Verification items for the finished model (mm, model axes). A direction names the side the tool comes from. Give positions to 0.01 mm unless a question says otherwise; leave off trailing zeros. Write each loop counter-clockwise with the first axis right and the second up, starting at its lowest first coordinate (ties: lowest second). Pieces come first, ordered by that corner, then holes.
from build123d import *

# Parameters (mm, degrees)
SKETCH1_W                                      = 223.52
SKETCH1_H                                      = 50.8
SKETCH1_R                                      = 3.2385
BOSS_EXTRUDE1_DEPTH                            = 6.858
SKETCH2_W                                      = 20
SKETCH2_H                                      = 6.35
BOSS_EXTRUDE2_DEPTH                            = 17.78
SKETCH3_R                                      = 2.25
CUT_EXTRUDE1_DEPTH                             = 17.78
SKETCH4_W                                      = 2.54
SKETCH4_H                                      = 17.78
BOSS_EXTRUDE3_DEPTH                            = 17.78
CUT_EXTRUDE2_DEPTH                             = 20
LPATTERN1_COUNT                                = 2
LPATTERN1_PITCH                                = 101.76
BOSS_EXTRUDE4_DEPTH                            = 2.54
CSK_FOR_6_FLAT_HEAD_MACHINE_SCREW1_D           = 3.7973
CSK_FOR_6_FLAT_HEAD_MACHINE_SCREW1_CSINK_D     = 7.9697834
CSK_FOR_6_FLAT_HEAD_MACHINE_SCREW1_CSINK_ANGLE = 82


with BuildPart() as part:
    # Sketch1 → Boss-Extrude1 (new body)
    with BuildSketch(Plane.XY):
        Rectangle(SKETCH1_W, SKETCH1_H)
        with Locations((-54.61, 6.35)):
            Circle(SKETCH1_R, mode=Mode.SUBTRACT)
        with Locations((54.61, 6.35)):
            Circle(SKETCH1_R, mode=Mode.SUBTRACT)
    extrude(amount=BOSS_EXTRUDE1_DEPTH)

    # Sketch2 → Boss-Extrude2 (add)
    with BuildSketch(Plane.XY.offset(6.858)):
        with Locations((-101.76, -22.225)):
            Rectangle(SKETCH2_W, SKETCH2_H)
    boss_extrude2 = extrude(amount=BOSS_EXTRUDE2_DEPTH)

    # Sketch3 → Cut-Extrude1 (cut)
    with BuildSketch(Plane(origin=(0, -19.05, 0), x_dir=(1, 0, 0), z_dir=(0, 1, 0))):
        with Locations((-101.76, -15.748)):
            Circle(SKETCH3_R)
    cut_extrude1 = extrude(amount=-CUT_EXTRUDE1_DEPTH, mode=Mode.SUBTRACT)

    # Sketch4 → Boss-Extrude3 (add)
    with BuildSketch(Plane(origin=(0, -19.05, 0), x_dir=(1, 0, 0), z_dir=(0, 1, 0))):
        with Locations((-110.49, -15.748)):
            Rectangle(SKETCH4_W, SKETCH4_H)
        with Locations((-93.03, -15.748)):
            Rectangle(SKETCH4_W, SKETCH4_H)
    boss_extrude3 = extrude(amount=BOSS_EXTRUDE3_DEPTH)

    # Sketch6 → Cut-Extrude2 (cut)
    with BuildSketch(Plane.ZY.offset(111.76)):
        Polygon((24.638, -1.27), (6.858, -1.27), (24.638, -19.05), align=None)
    cut_extrude2 = extrude(amount=-CUT_EXTRUDE2_DEPTH, mode=Mode.SUBTRACT)

    # LPattern1: Boss-Extrude2, Cut-Extrude1, Boss-Extrude3, Cut-Extrude2 ×2
    with Locations(*[(i * LPATTERN1_PITCH, 0, 0) for i in range(1, LPATTERN1_COUNT)]):
        add(boss_extrude2)
        add(cut_extrude1, mode=Mode.SUBTRACT)
        add(boss_extrude3)
        add(cut_extrude2, mode=Mode.SUBTRACT)

    # Sketch7 → Boss-Extrude4 (add)
    with BuildSketch(Plane.ZY.offset(111.76)):
        Polygon((24.638, -19.05), (24.638, 25.4), (6.858, 25.4), (6.858, -1.27), align=None)
    extrude(amount=-BOSS_EXTRUDE4_DEPTH)

    # CSK for #6 Flat Head Machine Screw1 (through all)
    with Locations(Plane(origin=(0, 0, 0), x_dir=(-1, 0, 0), z_dir=(0, 0, -1))):
        with Locations((-105.41, 12.7), (-105.41, -12.7)):
            CounterSinkHole(CSK_FOR_6_FLAT_HEAD_MACHINE_SCREW1_D / 2, CSK_FOR_6_FLAT_HEAD_MACHINE_SCREW1_CSINK_D / 2, counter_sink_angle=CSK_FOR_6_FLAT_HEAD_MACHINE_SCREW1_CSINK_ANGLE)


solid = part.part
Item 1: Sectioned sample at D-D on z = 10.25. Record the cut outline in (x, y).
Answer key:
outline: (-111.76, -25.4) - (-91.76, -25.4) - (-91.76, -4.66) - (-94.3, -4.66) - (-94.3, -19.05) - (-109.22, -19.05) - (-109.22, 25.4) - (-111.76, 25.4) - close; (-10, -25.4) - (10, -25.4) - (10, -4.66) - (7.46, -4.66) - (7.46, -19.05) - (-7.46, -19.05) - (-7.46, -4.66) - (-10, -4.66) - close
Item 2: Scan lines: line 1 along Y through (x, z) = (105.41, 3.8); line 2 along X through (y, z) = (-13, 13.5); line 3 along Y through (x, z) = (-54.61, 4.25). Record each from-to range of solid material in increasing order.
Answer key:
line 1: y = -25.4 to -14.6, -10.8 to 10.8, 14.6 to 25.4
line 2: x = -111.76 to -109.22, -94.3 to -91.76, -10 to -7.46, 7.46 to 10
line 3: y = -25.4 to 3.11, 9.59 to 25.4
Item 3: Set-up check for faces 1 (the face through (-10, -16, 14)), 2 (the face through (-100, -19.05, 18)), 3 (the face through (111.76, 0, 3)): record each of +Z, -Z, +X, -X, +Y, -Y from which the full face is reachable in a straight line by a thin tool's end or side.
Answer key:
face 1: +Z, +Y, -Y
face 2: +Z, +Y
face 3: +Z, -Z, +X, +Y, -Y
Item 4: Depth check by flat-ended pin: pin 1 (6 mm diameter, centred on x = 50.5, y = 14.5, fed in from -Z); pin 2 (1 mm diameter, centred on x = -63, y = 17, fed in from +Z); pin 3 (14 mm diameter, centred on y = 10, z = 17, fed in from +X); pin 4 (5.5 mm diameter, centred on y = -11.5, z = 18.5, fed in from +X). Enter the tip coordinate at first touch or a pass-through.
Answer key:
pin 1: stops at z = 0
pin 2: stops at z = 6.86
pin 3: stops at x = -109.22
pin 4: stops at x = 10
Item 5: Sectioned sample at C-C on x = 105.41. Record the cut outline in (y, z).
Answer key:
outline: (-25.4, 0) - (-16.68, 0) - (-14.6, 2.4) - (-14.6, 6.86) - (-25.4, 6.86) - close; (-10.8, 2.4) - (-8.72, 0) - (8.72, 0) - (10.8, 2.4) - (10.8, 6.86) - (-10.8, 6.86) - close; (14.6, 2.4) - (16.68, 0) - (25.4, 0) - (25.4, 6.86) - (14.6, 6.86) - close
Item 6: Release check for a two-part mould opening along Z. For faces 4 (the face through (7.46, -14, 12)), 5 (the face through (-0.293, -22.181, 13.517)), 6 (the face through (-93.048, -10.036, 15.624)), 7 (the face through (-2, 0, 0)) record: released by +Z, released by -Z, zero draft, split by the parting line, or undercut.
Answer key:
face 4: zero draft
face 5: undercut
face 6: released by +Z
face 7: released by -Z
Item 7: Sectioned sample at B-B on x = -54.61. Record the cut outline in (y, z).
Answer key:
outline: (-25.4, 0) - (3.11, 0) - (3.11, 6.86) - (-25.4, 6.86) - close; (9.59, 0) - (25.4, 0) - (25.4, 6.86) - (9.59, 6.86) - close
Item 8: Sectioned sample at A-A on y = 12.7. Record the cut outline in (x, z).
Answer key:
outline: (-111.76, 0) - (101.43, 0) - (103.51, 2.4) - (103.51, 6.86) - (-109.22, 6.86) - (-109.22, 24.64) - (-111.76, 24.64) - close; (107.31, 2.4) - (109.39, 0) - (111.76, 0) - (111.76, 6.86) - (107.31, 6.86) - close
